Model file for the job. Use its own axes, mm. A direction names the side the tool comes from. Round coordinates to 2 decimals unless told otherwise and drop trailing zeros. Loops run counter-clockwise (first coordinate to the right, second up) from the corner with the lowest first, then second, coordinate; pieces in that order, holes last. Notation, with made-up numbers: M 29,67.25 L 82,67.25 A28 ccw 82,91.25 Z; hole C 72.25,21 d1. An arc over 180 degrees is marked long. Use a Markdown table: item, result. Add a question column.
Item 1: Wall check: L1, parallel to X at y = 21, z = -13.5; L2, parallel to Y at x = 22.5, z = 5; L3, parallel to X at y = 23, z = -6.5. Give the ranges that are in metal, low to high. Write a range as from..to.
Item 2: Saw through at A-A on y = 23. Write the cut outline in (x, z).
Item 3: Saw through at C-C on z = -9. Write the cut outline in (x, y).
Item 4: Saw through at D-D on y = 13.5. Write the cut outline in (x, z), then the cut area to 3 significant figures.
Item 5: Saw through at B-B on x = -18. Write the cut outline in (y, z).
Item 6: Tool access for faces 1 (the flat face through (0, 22, 0)), 2 (the flat face through (0, 0, 0)), 3 (the cylindrical face through (38.776, 1.816, 2.168)): list every direction of +Z, -Z, +X, -X, +Y, -Y with a clear straight run to the whole face (end or side of a thin tool).
Item 7: Pin check, flat tips, straight feed: P1, Ø5.5, axis at x = 15.5, z = 9.5, coming from the +Y side; P2, Ø2, axis at x = 2.5, z = 0, coming from the +Y side; P3, Ø1, axis at x = -10, y = 28, coming from the +Z side. Stop position of each tip, or through.
Item 8: Two-plate mould, pull along Z, no slides. Class faces 4 (the cylindrical face through (18.233, 23.479, 10.341)), 5 (the flat face through (-23, 11, 0)), 6 (the flat face through (0, 11, -16)): +Z half, -Z half, draft (parallel to the pull), parting line (faces both ways), or undercut.
```python
from build123d import *

# Parameters (mm, degrees)
SKETCH1_W           = 46
SKETCH1_H           = 32
BOSS_EXTRUDE1_DEPTH = 22
SKETCH3_R           = 10
BOSS_EXTRUDE3_DEPTH = 32
SKETCH4_R           = 3
BOSS_EXTRUDE4_DEPTH = 17
SKETCH5_R           = 3.5
BOSS_EXTRUDE6_DEPTH = 3


with BuildPart() as part:
    # Sketch1 → Boss-Extrude1 (new body)
    with BuildSketch(Plane(origin=(0, 0, 0), x_dir=(1, 0, 0), z_dir=(0, 1, 0))):
        Rectangle(SKETCH1_W, SKETCH1_H)
    extrude(amount=BOSS_EXTRUDE1_DEPTH)

    # Sketch3 → Boss-Extrude3 (add)
    with BuildSketch(Plane(origin=(23, 0, 0), x_dir=(0, 0, -1), z_dir=(1, 0, 0))):
        with Locations((0, 11.57774751)):
            Circle(SKETCH3_R)
    extrude(amount=BOSS_EXTRUDE3_DEPTH)

    # Sketch4 → Boss-Extrude4 (add)
    with BuildSketch(Plane(origin=(0, 22, 0), x_dir=(1, 0, 0), z_dir=(0, 1, 0))):
        with Locations((-9, 0)):
            Circle(SKETCH4_R)
    extrude(amount=BOSS_EXTRUDE4_DEPTH)

    # Sketch5 → Boss-Extrude6 (add)
    with BuildSketch(Plane(origin=(0, 22, 0), x_dir=(1, 0, 0), z_dir=(0, 1, 0))):
        with Locations((-18, -9)):
            Circle(SKETCH5_R)
        with Locations((15, 9)):
            Circle(SKETCH5_R)
        with Locations((15, -9)):
            Circle(SKETCH5_R)
        with Locations((-18, 9)):
            Circle(SKETCH5_R)
    extrude(amount=BOSS_EXTRUDE6_DEPTH)


solid = part.part
```
Entries:
| question | item | result |
|---|---|---|
| 1 | L1 | -23..23 |
| 1 | L2 | 0..22 |
| 1 | L3 | -20.45..-15.55, 12.55..17.45 |
| 2 | outline | C -18,-9 d7; C -18,9 d7; C -9,0 d6; C 15,-9 d7; C 15,9 d7 |
| 3 | outline | M -23,0 L 23,0 L 23,7.22 L 55,7.22 L 55,15.94 L 23,15.94 L 23,22 L 18.5,22 L 18.5,25 L 11.5,25 L 11.5,22 L -14.5,22 L -14.5,25 L -21.5,25 L -21.5,22 L -23,22 Z |
| 4 | outline | M -23,-16 L 23,-16 L 23,-9.81 L 55,-9.81 L 55,9.81 L 23,9.81 L 23,16 L -23,16 Z |
| 4 | area | 2,100 mm2 |
| 5 | outline | M 0,-16 L 22,-16 L 22,-12.5 L 25,-12.5 L 25,-5.5 L 22,-5.5 L 22,5.5 L 25,5.5 L 25,12.5 L 22,12.5 L 22,16 L 0,16 Z |
| 6 | face 1 | +Y |
| 6 | face 2 | +Z, -Z, +X, -X, -Y |
| 6 | face 3 | +X |
| 7 | P1 | y = 25 |
| 7 | P2 | y = 22 |
| 7 | P3 | z = 2.96 |
| 8 | face 4 | undercut |
| 8 | face 5 | draft |
| 8 | face 6 | -Z half |
